from build123d import *

# Parameters (mm, degrees)
F0_R           = 175
F0_R_2         = 1.65
F1_DEPTH       = 8
F3_D           = 4.4
F3_CSINK_D     = 8.96
F3_CSINK_ANGLE = 90


with BuildPart() as f1:
    # F0 (on Top) → F1 (new body)
    with BuildSketch(Plane.XY):
        Circle(F0_R)
        with Locations((-144.2451912543, -83.28)):
            Circle(F0_R_2, mode=Mode.SUBTRACT)
        with Locations((0, -166.56)):
            Circle(F0_R_2, mode=Mode.SUBTRACT)
        with Locations((144.2451912543, -83.28)):
            Circle(F0_R_2, mode=Mode.SUBTRACT)
        with Locations((-144.2451912543, 83.28)):
            Circle(F0_R_2, mode=Mode.SUBTRACT)
        with Locations((144.2451912543, 83.28)):
            Circle(F0_R_2, mode=Mode.SUBTRACT)
        with Locations((0, 166.56)):
            Circle(F0_R_2, mode=Mode.SUBTRACT)
    extrude(amount=F1_DEPTH)

    # F3 (through all)
    with Locations(Plane.XY.offset(8)):
        with Locations((-144.2451912543, -83.28), (-144.2451912543, 83.28), (0, 166.56), (144.2451912543, 83.28), (144.2451912543, -83.28), (0, -166.56)):
            CounterSinkHole(F3_D / 2, F3_CSINK_D / 2, counter_sink_angle=F3_CSINK_ANGLE)


solid = f1.part
For this review, take the finished solid that the model builds, in its own axes (mm). Round coordinates to 2 decimals unless told otherwise and drop trailing zeros. Order: outer loops, then holes, each group sorted by start corner. A loop starts at its lowest first (then second) coordinate and runs counter-clockwise, first axis right, second up. Notation, with made-up numbers: M -3,62 L 43,62 A20 cw 43,85 Z; hole C 62,65 d5. An arc over 180 degrees is marked long. Use a Markdown table: item, result. Add a question column.
Item 1: Insertion check: pin 1 (2.5 mm diameter, centred on x = 0, y = 166.56, fed in from -Z); pin 2 (3 mm diameter, centred on x = 68.5, z = 4, fed in from +Y); pin 3 (5 mm diameter, centred on x = -144.25, y = 83.28, fed in from +Z); pin 4 (1 mm diameter, centred on x = 79, z = 3, fed in from -Y). Each pin has a flat end and moves straight along its axis. Give the tip position at first contact, or say it passes through.
Item 2: Add section B-B, the plane y = 52. Give the boundary of the cut face in (x, z).
Item 3: Add section C-C, the plane x = 42. Give the boundary of the cut face in (y, z).
Item 4: Mouldability with a two-part tool opening along X and no side actions: class faces 1 (the cylindrical face through (-128.982, 118.273, 3.944)), 2 (the conical face through (1.83, -167.97, 5.83)), 3 (the flat face through (-2, 2, 8)) as released by +X, released by -X, zero draft, split by the parting line, or undercut.
Item 5: To check wall thickness, follow line 1 along Y through (x, z) = (0, 2.95); line 2 along X through (y, z) = (83.28, 1.8); line 3 along Y through (x, z) = (105.5, 4.75). State the ranges of each line that lie inside material, in increasing order.
Item 6: Add section A-A, the plane z = 1.5. Give the boundary of the cut face in (x, y).
Geometry results:
| question | item | result |
|---|---|---|
| 1 | pin 1 | passes through |
| 1 | pin 2 | stops at y = 161.67 |
| 1 | pin 3 | stops at z = 6.02 |
| 1 | pin 4 | stops at y = -156.41 |
| 2 | outline | M -167.1,0 L 167.1,0 L 167.1,8 L -167.1,8 Z |
| 3 | outline | M -169.89,0 L 169.89,0 L 169.89,8 L -169.89,8 Z |
| 4 | face 1 | split by the parting line |
| 4 | face 2 | undercut |
| 4 | face 3 | zero draft |
| 5 | line 1 | y = -175 to -168.76, -164.36 to 164.36, 168.76 to 175 |
| 5 | line 2 | x = -153.91 to -146.45, -142.05 to 142.05, 146.45 to 153.91 |
| 5 | line 3 | y = -139.62 to 139.62 |
| 6 | outline | C 0,0 d350; hole C -144.25,-83.28 d4.4; hole C -144.25,83.28 d4.4; hole C 0,-166.56 d4.4; hole C 0,166.56 d4.4; hole C 144.25,-83.28 d4.4; hole C 144.25,83.28 d4.4 |
